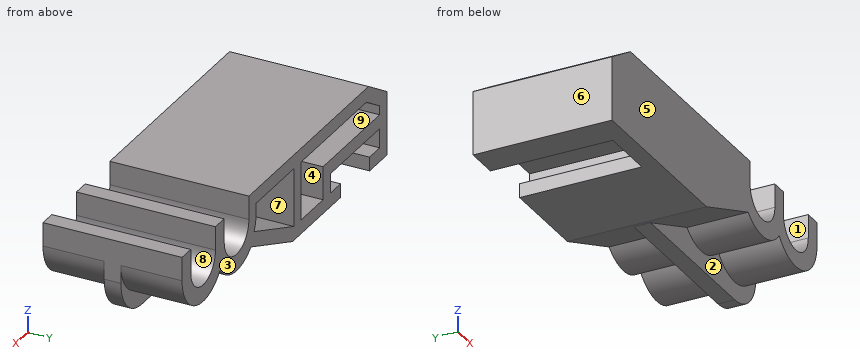
```python
from build123d import *

# Parameters (mm, degrees)
BOSS_EXTRUDE1_DEPTH = 10
BOSS_EXTRUDE2_DEPTH = 10
CUT_EXTRUDE1_DEPTH  = 10
SHELL2_T            = -1
SKETCH4_W           = 1
SKETCH4_H           = 4.2
BOSS_EXTRUDE3_DEPTH = 9
SKETCH7_W           = 6.8
SKETCH7_H           = 1
BOSS_EXTRUDE4_DEPTH = 9
SKETCH8_W           = 4
SKETCH8_H           = 1
CUT_EXTRUDE2_DEPTH  = 8.8
BOSS_EXTRUDE5_DEPTH = 0.6


with BuildPart() as part:
    # Sketch1 → Boss-Extrude1 (new body)
    with BuildSketch(Plane(origin=(0, 0, 0), x_dir=(1, 0, 0), z_dir=(0, 1, 0))):
        with BuildLine():
            ThreePointArc((-2.9, 0), (-0.932737905, 2.745906044), (2.3, 1.766352173))
            ThreePointArc((2.3, 1.766352173), (5.532737905, 2.745906044), (7.5, 0))
            Line((7.5, 0), (7.5, -1.7))
            Line((7.5, -1.7), (6.3, -1.7))
            Line((6.3, -1.7), (6.3, 0))
            ThreePointArc((6.3, 0), (4.6, 1.7), (2.9, 0))
            Line((2.9, 0), (2.9, -1.7))
            Line((2.9, -1.7), (1.7, -1.7))
            Line((1.7, -1.7), (1.7, 0))
            ThreePointArc((1.7, 0), (0, 1.7), (-1.7, 0))
            Line((-1.7, 0), (-1.7, -1.7))
            Line((-1.7, -1.7), (-2.9, -1.7))
            Line((-2.9, -1.7), (-2.9, 0))
        make_face()
    extrude(amount=BOSS_EXTRUDE1_DEPTH)

    # Sketch2 → Boss-Extrude2 (add)
    with BuildSketch(Plane.XZ):
        with BuildLine():
            Line((-2.9, 1.7), (-20.7, 1.7))
            Line((-20.7, 1.7), (-20.7, -4.5))
            Line((-20.7, -4.5), (-7.7, -4.5))
            Line((-7.7, -4.5), (-1.972618929, -2.125740944))
            ThreePointArc((-1.972618929, -2.125740944), (-2.658062724, -1.159613105), (-2.9, 0))
            Line((-2.9, 0), (-2.9, 1.7))
        make_face()
    extrude(amount=-BOSS_EXTRUDE2_DEPTH)

    # Sketch3 → Cut-Extrude1 (cut)
    with BuildSketch(Plane.XZ):
        Polygon((-18.162284492, 1.7), (-20.7, 0.1), (-20.7, 1.7), align=None)
    extrude(amount=-CUT_EXTRUDE1_DEPTH, mode=Mode.SUBTRACT)

    # Shell2
    shell2_openings = [part.faces().sort_by_distance(p)[0] for p in [
        (-2.051423917, 10, -0.549910722),
    ]]
    offset(amount=SHELL2_T, openings=shell2_openings, kind=Kind.INTERSECTION)

    # Sketch4 → Boss-Extrude3 (add)
    with BuildSketch(Plane(origin=(0, 1, 0), x_dir=(1, 0, 0), z_dir=(0, 1, 0))):
        with Locations((-8.399059546, 1.4)):
            Rectangle(SKETCH4_W, SKETCH4_H)
    extrude(amount=BOSS_EXTRUDE3_DEPTH)

    # Sketch7 → Boss-Extrude4 (add)
    with BuildSketch(Plane(origin=(0, 1, 0), x_dir=(1, 0, 0), z_dir=(0, 1, 0))):
        with Locations((-16.3, 1.6)):
            Rectangle(SKETCH7_W, SKETCH7_H)
        Polygon((-11.9, 3.5), (-12.9, 3.5), (-12.9, 2.1), (-12.9, 1.1), (-11.9, 1.1), align=None)
    extrude(amount=BOSS_EXTRUDE4_DEPTH)

    # Sketch8 → Cut-Extrude2 (cut)
    with BuildSketch(Plane(origin=(0, 10, 0), x_dir=(1, 0, 0), z_dir=(0, 1, 0))):
        with Locations((-16.3, 4)):
            Rectangle(SKETCH8_W, SKETCH8_H)
    extrude(amount=-CUT_EXTRUDE2_DEPTH, mode=Mode.SUBTRACT)

    # Sketch9 → Boss-Extrude5 (add, symmetric)
    with BuildSketch(Plane(origin=(0, 5, 0), x_dir=(1, 0, 0), z_dir=(0, 1, 0))):
        with BuildLine():
            Line((0, 4.2), (-6.976315566, 4.2))
            Line((-6.976315566, 4.2), (-1.972618929, 2.125740944))
            ThreePointArc((-1.972618929, 2.125740944), (0.243073371, 2.889795034), (2.3, 1.766352173))
            ThreePointArc((2.3, 1.766352173), (5.532737905, 2.745906044), (7.5, 0))
            Line((7.5, 0), (7.5, 1.299833538))
            ThreePointArc((7.5, 1.299833538), (6.65066852, 3.350550812), (4.6, 4.2))
            Line((4.6, 4.2), (0, 4.2))
        make_face()
    extrude(amount=BOSS_EXTRUDE5_DEPTH, both=True)


solid = part.part
```
Design review of the part built by this model. Coordinates are the model's own, in mm. Face numbers are marked on the shaded views. A direction names the side the tool comes from. Give positions to 0.01 mm unless a question says otherwise; leave off trailing zeros. Order: outer loops, then holes, each group sorted by start corner. A loop starts at its lowest first (then second) coordinate and runs counter-clockwise, first axis right, second up. Notation, with made-up numbers: (-18, 71) -> (2, 71) arc R6 ccw to (2, 82) -> close; hole circle Ø3 at (-8.75, 24). An arc over 180 degrees is marked (long way). Write item = value, one per line. Start each with the question number.
(1) We need section A-A on x = -9.75. Write out the cut boundary in (y, z), plus the area to 3 significant figures.
(2) We need section C-C on x = -5.25. Write out the cut boundary in (y, z), plus the area to 3 significant figures.
(3) We need section B-B on y = 3. State how many separate pieces and enclosed holes the cut face has, plus the area to 3 significant figures.
(4) Mouldability with a two-part tool opening along Z and no side actions: class the marked faces 6, 7, 8 and 9 as +Z half, -Z half, draft (parallel to the pull), parting line (faces both ways), or undercut.
(5) We need section D-D on x = 0. Write out the cut boundary in (y, z), plus the area to 3 significant figures.
(6) For pin 1 (0.8 mm diameter, centred on y = 7, z = 1, fed in from -X); pin 2 (2 mm diameter, centred on x = 4.5, y = 2.5, fed in from +Z); pin 3 (0.6 mm diameter, centred on x = -2, y = 5, fed in from -Z), all flat-tipped, find the tip position at first contact; note any pin that passes through.
(7) For the marked faces 1, 2, 3, 4 and 5, list the 3-axis set-ups (+Z, -Z, +X, -X, +Y, -Y) from which the entire face can be reached by the end or side of a thin tool; tool diameter is ignored.
(8) To check wall thickness, follow line 1 along Z through (x, y) = (-13.25, 7.25); line 2 along X through (y, z) = (7, -3.25); line 3 along X through (y, z) = (8.5, -1). State the ranges of each line that lie inside material, in increasing order.
Numbers:
q1.outline = (0, -4.5) -> (10, -4.5) -> (10, -3.5) -> (1, -3.5) -> (1, 0.7) -> (10, 0.7) -> (10, 1.7) -> (0, 1.7) -> close
q1.area = 24.2 mm^2
q2.outline = (0, -3.48) -> (4.4, -3.48) -> (4.4, -4.2) -> (5.6, -4.2) -> (5.6, -3.48) -> (10, -3.48) -> (10, -2.4) -> (1, -2.4) -> (1, 0.7) -> (10, 0.7) -> (10, 1.7) -> (0, 1.7) -> close
q2.area = 24.8 mm^2
q3.separate_pieces = 1
q3.enclosed_holes = 2
q3.area = 70.9 mm^2
q4.face_6 = draft
q4.face_7 = undercut
q4.face_8 = +Z half
q4.face_9 = undercut
q5.outline = (0, -2.9) -> (4.4, -2.9) -> (4.4, -4.2) -> (5.6, -4.2) -> (5.6, -2.9) -> (10, -2.9) -> (10, -1.7) -> (0, -1.7) -> close
q5.area = 13.6 mm^2
q6.pin_1 = -19.91
q6.pin_2 = -1.3
q6.pin_3 = -4.2
q7.face_1 = +Z, +Y, -Y
q7.face_2 = -Z, -Y
q7.face_3 = +Z, -Z, +X, -X, +Y
q7.face_4 = +Y
q7.face_5 = +Z, -Z, +X, -X, -Y
q8.line_1 = -4.5 to -3.5, -2.1 to -1.1, 0.7 to 1.7
q8.line_2 = -20.7 to -19.7, -12.9 to -11.9, -8.9 to -7.9, -7.3 to -4.68
q8.line_3 = -20.7 to -19.7, -8.9 to -7.9, -2.51 to -1.37, 1.37 to 3.23, 5.97 to 7.32
